from build123d import *

# Parameters (mm, degrees)
SKETCH2_OUTSIDE_W  = 23.078
SKETCH2_OUTSIDE_H  = 23.078
CUT_EXTRUDE1_DEPTH = 17.136867678
SKETCH4_W          = 1
SKETCH4_H          = 1
CUT_EXTRUDE2_DEPTH = 1


with BuildPart() as part:
    # Sketch1 → Revolve1 (revolve)
    with BuildSketch(Plane.XY, mode=Mode.PRIVATE) as revolve1_sk:
        Polygon((-7.506454643, 8), (-4.506454643, 8), (0, 0.5), (0, 0.2), (-0.5, 0.2), (-0.980688495, 1), (-8.506454643, 1), (-8.897014045, 1.65), (-11.506454643, 1.65), (-11.506454643, 2.45), (-7.506454643, 2.45), align=None)
    revolve(revolve1_sk.sketch.rotate(Axis((-1000, 0, 0), (1, 0, 0)), 90), axis=Axis((-1000, 0, 0), (1, 0, 0)))

    # Sketch2 outside → Cut-Extrude1 (cut, through all)
    with BuildSketch(Plane(origin=(0, 0, 0), x_dir=(0, 0, -1), z_dir=(1, 0, 0))):
        Rectangle(SKETCH2_OUTSIDE_W, SKETCH2_OUTSIDE_H)
        Polygon((4.618802154, 0), (2.309401077, 4), (-2.309401077, 4), (-4.618802154, 0), (-2.309401077, -4), (2.309401077, -4), align=None, mode=Mode.SUBTRACT)
    extrude(amount=-CUT_EXTRUDE1_DEPTH, mode=Mode.SUBTRACT)

    # Sketch3 → Cut-Revolve1 (revolve, cut)
    with BuildSketch(Plane(origin=(0, 0, 0), x_dir=(1, 0, 0), z_dir=(0, 1, 0)), mode=Mode.PRIVATE) as cut_revolve1_sk:
        Polygon((-10.36359318, -4.026237068), (-10.163897775, -5.158765984), (-2.285435751, -3.769580562), (-1.80463913, -2.517062542), align=None)
    revolve(cut_revolve1_sk.sketch.rotate(Axis((-1.80463913, 0, 2.517062542), (-0.9848077530122068, 0, 0.17364817766693816)), 180), axis=Axis((-1.80463913, 0, 2.517062542), (-0.9848077530122068, 0, 0.17364817766693816)), mode=Mode.SUBTRACT)

    # Sketch4 → Cut-Extrude2 (cut)
    with BuildSketch(Plane.ZY.offset(7.506454643)):
        with Locations((4.118802154, 0)):
            Rectangle(SKETCH4_W, SKETCH4_H)
    extrude(amount=-CUT_EXTRUDE2_DEPTH, mode=Mode.SUBTRACT)


solid = part.part
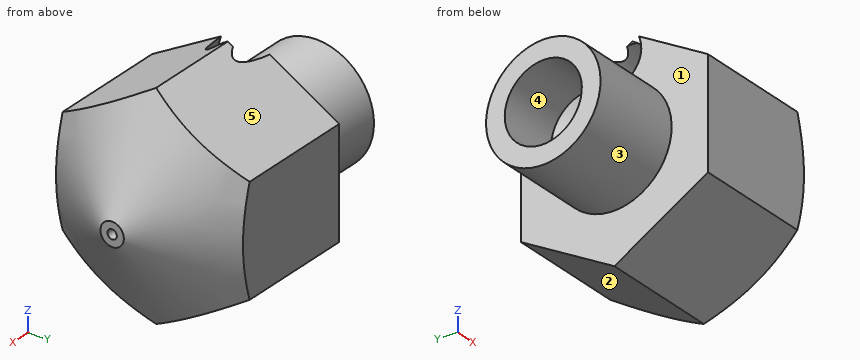
The listing builds one solid part. Answer for the finished solid, in the listing's coordinates (mm). Face numbers are marked on the shaded views. A direction names the side the tool comes from. Coordinates: 2 decimals unless noted, no trailing zeros. Loops run counter-clockwise (first coordinate to the right, second up) from the corner with the lowest first, then second, coordinate; pieces in that order, holes last.
1) Determine the mould class of the marked faces 3, 4 and 5 for opening direction Y: pulls with the +Y half, pulls with the -Y half, needs draft (parallel to the pull), parting line crosses it, or undercut.
2) Find section B-B on x = -1.5. Write down the section's boundary in (y, z).
3) Find the intervals of material crossed by L1, parallel to Z at x = -3.25, y = -0.5; L2, parallel to Y at x = -3, z = 0; L3, parallel to Y at x = -10.25, z = 0, in increasing order.
4) Flat-ended cylindrical pins translate along their axes: pin 1 Ø4 at (x, y) = (-3, 3) entering from -Z; pin 2 Ø2.5 at (y, z) = (0, 0) entering from -X; pin 3 Ø4 at (x, y) = (-9, 0.5) entering from +Z; pin 4 Ø4.5 at (y, z) = (0, 0) entering from -X. Find the tip coordinate at first contact, or state that the pin passes through.
5) A tool of negligible diameter and unlimited length cuts with its end or side. For the marked faces 1 and 2, from which of +Z, -Z, +X, -X, +Y, -Y can it reach the whole face along a straight path? Write none if from no direction.
6) Find section A-A on z = 0. Write down the section's boundary in (x, y).
Values:
1. face 3: parting line crosses it
1. face 4: undercut
1. face 5: pulls with the +Y half
2. outline: circle Ø5.99 at (0, 0); hole circle Ø2 at (0, 0)
3. L1: z = -4.33 to -0.87, 0.87 to 1.72, 3.82 to 4.33
3. L2: y = -4 to -1, 1 to 4
3. L3: y = -2.45 to -1.65, 1.65 to 2.45
4. pin 1: stops at z = -4.04
4. pin 2: stops at x = -8.66
4. pin 3: stops at z = 4.05
4. pin 4: stops at x = -11.51
5. face 1: -X
5. face 2: -Z, +X, -X, +Y
6. outline: (-11.51, -2.45) - (-7.51, -2.45) - (-7.51, -4) - (-2.1, -4) - (0, -0.5) - (0, -0.2) - (-0.5, -0.2) - (-0.98, -1) - (-8.51, -1) - (-8.9, -1.65) - (-11.51, -1.65) - close; (-11.51, 1.65) - (-8.9, 1.65) - (-8.51, 1) - (-0.98, 1) - (-0.5, 0.2) - (0, 0.2) - (0, 0.5) - (-2.1, 4) - (-7.51, 4) - (-7.51, 2.45) - (-11.51, 2.45) - close
